Here's how the part is built. I have some questions about the finished solid (model axes, mm). Coordinates: 2 decimals unless noted, no trailing zeros. Write each loop counter-clockwise with the first axis right and the second up, starting at its lowest first coordinate (ties: lowest second). Pieces come first, ordered by that corner, then holes. Notation, with made-up numbers: (84.25, -39) -> (142.25, -39) arc R34 ccw to (142.25, -9) -> close; hole circle Ø7 at (67, 78.5). An arc over 180 degrees is marked (long way). Use a Markdown table: item, result. Add a question column.
Item 1: Imagine slicing it at C-C, the plane y = -5.5. Write out the boundary of the cut face in (x, z).
Item 2: Imagine slicing it at B-B, the plane z = 0. Write out the boundary of the cut face in (x, y), and give its area (3 significant figures).
Item 3: Will these pins go through, and if not, where does the flat tip stop? pin 1 Ø3 at (x, y) = (2.5, 4) entering from +Z; pin 2 Ø1.5 at (y, z) = (1, 1) entering from -X; pin 3 Ø2 at (y, z) = (3.5, 2) entering from +X.
Item 4: If I drill on line 1 along Z through (x, y) = (0, -1.75); line 2 along X through (y, z) = (2, -0.25); line 3 along X through (y, z) = (4.75, 0.9), over which ranges is the centre line in solid material (lowest first)? Write a range as from..to.
Item 5: If we mould it in two halves opening along X, with no side actions, what happens to faces 1 (the cylindrical face through (3, 0, 0)), 2 (the flat face through (-1.3, -7.5, -2)), 3 (the cylindrical face through (1.438, -0.098, 0.748))? For each: pulls with the +X half, pulls with the -X half, needs draft (parallel to the pull), parting line crosses it, or undercut.
Item 6: Imagine slicing it at A-A, the plane x = 0. Write out the boundary of the cut face in (y, z), and give its area (3 significant figures).
Autodesk Inventor part; units mm, degrees
ref_plane "YZ Plane" through (0, 0, 0) normal (1, 0, 0) x (0, 1, 0)
ref_plane "XZ Plane" through (0, 0, 0) normal (0, 1, 0) x (-1, 0, 0)
ref_plane "XY Plane" through (0, 0, 0) normal (0, 0, 1) x (1, 0, 0)
sketch "Sketch1" plane through (0, 0, 0) normal (0, 1, 0) x (-1, 0, 0)
  circle A0 centre (0, 0) radius 3
  dimension "d0" = 6
extrude "Extrusion1" add sketch "Sketch1" along normal mid plane 15
sketch "Sketch2" plane through (0, 7.5, 0) normal (0, 1, 0) x (1, 0, 0)
  point P0 (0, 0)
  point P1 (0, 0)
hole "Hole1" at (0, 7.5, 0) direction (0, -1, 0) diameter 3.242 depth 15
chamfer "Chamfer1" distance 0.5 angle 45 2 edges at (0, 7.5, -1.621) (0, -7.5, -1.621)
properties part number "Standoff_GB"
Ans:
| question | item | result |
|---|---|---|
| 1 | outline | circle Ø6 at (0, 0); hole circle Ø3.24 at (0, 0) |
| 2 | outline | (-3, -7.5) -> (-2.12, -7.5) -> (-1.62, -7) -> (-1.62, 7) -> (-2.12, 7.5) -> (-3, 7.5) -> close; (1.62, -7) -> (2.12, -7.5) -> (3, -7.5) -> (3, 7.5) -> (2.12, 7.5) -> (1.62, 7) -> close |
| 2 | area | 40.9 mm^2 |
| 3 | pin 1 | stops at z = 2.83 |
| 3 | pin 2 | stops at x = -2.99 |
| 3 | pin 3 | stops at x = 2.83 |
| 4 | line 1 | z = -3..-1.62, 1.62..3 |
| 4 | line 2 | x = -2.99..-1.6, 1.6..2.99 |
| 4 | line 3 | x = -2.86..-1.35, 1.35..2.86 |
| 5 | face 1 | parting line crosses it |
| 5 | face 2 | needs draft |
| 5 | face 3 | undercut |
| 6 | outline | (-7.5, -3) -> (7.5, -3) -> (7.5, -2.12) -> (7, -1.62) -> (-7, -1.62) -> (-7.5, -2.12) -> close; (-7.5, 2.12) -> (-7, 1.62) -> (7, 1.62) -> (7.5, 2.12) -> (7.5, 3) -> (-7.5, 3) -> close |
| 6 | area | 40.9 mm^2 |
